Read the model definition and answer for the solid it produces. Units are mm, in the model's axes. A direction names the side the tool comes from. Give positions to 0.01 mm unless a question says otherwise; leave off trailing zeros. Loops run counter-clockwise (first coordinate to the right, second up) from the corner with the lowest first, then second, coordinate; pieces in that order, holes last. Notation, with made-up numbers: (-20, 48.25) - (16, 48.25) arc R26 ccw to (16, 80.25) - close; hole circle Ø7 at (-8.75, 86.5). An arc over 180 degrees is marked (long way). Use a Markdown table: item, result. Add a question column.
Item 1: For a pull along Y with two mould halves and no side action, classify faces 4 (the face through (12, 0, 26)), 5 (the face through (4.87, -6.51, 14.34)), 6 (the face through (-3.3, -0.6, 14.3)) as +Y half, -Y half, draft (parallel to the pull), parting line (faces both ways), or undercut.
Item 2: Which of the six approach directions +Z, -Z, +X, -X, +Y, -Y give full straight-line access (tool end or side, diameter ignored) to faces 1 (the face through (4.87, 8.49, 14.34)), 2 (the face through (15, 0, -12)), 3 (the face through (5, -7, 26))?
Item 3: A cutting plane is placed at B-B (x = 12.5). Determine the outline of the cut face in (y, z).
Item 4: Each of these flat-tipped pins is pushed along its axis until it touches: P1, Ø2, axis at x = -2.5, y = 4.5, coming from the +Z side; P2, Ø3, axis at y = 1, z = 17.5, coming from the -X side; P3, Ø8, axis at y = -8, z = 12.5, coming from the +X side. Where does it stop, or does it pass through?
Item 5: A cutting plane is placed at C-C (z = -14.5). Determine the outline of the cut face in (x, y).
Item 6: A cutting plane is placed at A-A (z = 8.5). Determine the outline of the cut face in (x, y), plus the area to 3 significant figures.
Item 7: Consider probe 1 along X at (y, z) = (6.75, -9.5); probe 2 along Y at (x, z) = (-4.25, -2.5); probe 3 along Z at (x, y) = (2.25, -7.25). Determine where each line is inside the solid, lowest interval first. Write a range as [from, to].
Item 8: A cutting plane is placed at D-D (y = 0). Determine the outline of the cut face in (x, z), plus the area to 3 significant figures.
from build123d import *

# Parameters (mm, degrees)
SKETCH1_W           = 26
SKETCH1_H           = 21
SKETCH1_W_2         = 20
SKETCH1_H_2         = 15
BOSS_EXTRUDE1_DEPTH = 25
SKETCH2_W           = 26
SKETCH2_H           = 21
BOSS_EXTRUDE2_DEPTH = 3
SKETCH3_R           = 1
BOSS_EXTRUDE3_DEPTH = 23


with BuildPart() as part:
    # Sketch1 → Boss-Extrude1 (new body)
    with BuildSketch(Plane.XY):
        with Locations((5, 0)):
            Rectangle(SKETCH1_W, SKETCH1_H)
        with Locations((5, 0)):
            Rectangle(SKETCH1_W_2, SKETCH1_H_2, mode=Mode.SUBTRACT)
    extrude(amount=-BOSS_EXTRUDE1_DEPTH)

    # Sketch2 → Boss-Extrude2 (add)
    with BuildSketch(Plane.XY):
        with Locations((5, 0)):
            Rectangle(SKETCH2_W, SKETCH2_H)
    extrude(amount=BOSS_EXTRUDE2_DEPTH)

    # Sketch3 → Boss-Extrude3 (add)
    with BuildSketch(Plane.XY.offset(3)):
        with Locations((12.5, 0)):
            Circle(SKETCH3_R)
        with Locations((5, -7.5)):
            Circle(SKETCH3_R)
        with Locations((-2.5, 0)):
            Circle(SKETCH3_R)
        with Locations((5, 7.5)):
            Circle(SKETCH3_R)
    extrude(amount=BOSS_EXTRUDE3_DEPTH)


solid = part.part
Geometry says:
| question | item | result |
|---|---|---|
| 1 | face 4 | draft |
| 1 | face 5 | undercut |
| 1 | face 6 | parting line |
| 2 | face 1 | +Z |
| 2 | face 2 | -Z |
| 2 | face 3 | +Z, +X, -X, +Y, -Y |
| 3 | outline | (-10.5, -25) - (-7.5, -25) - (-7.5, 0) - (7.5, 0) - (7.5, -25) - (10.5, -25) - (10.5, 3) - (1, 3) - (1, 26) - (-1, 26) - (-1, 3) - (-10.5, 3) - close |
| 4 | P1 | z = 3 |
| 4 | P2 | x = -3.5 |
| 4 | P3 | x = 6 |
| 5 | outline | (-8, -10.5) - (18, -10.5) - (18, 10.5) - (-8, 10.5) - close; hole (-5, -7.5) - (15, -7.5) - (15, 7.5) - (-5, 7.5) - close |
| 6 | outline | circle Ø2 at (-2.5, 0); circle Ø2 at (5, -7.5); circle Ø2 at (5, 7.5); circle Ø2 at (12.5, 0) |
| 6 | area | 12.6 mm² |
| 7 | probe 1 | [-8, -5], [15, 18] |
| 7 | probe 2 | [-10.5, -7.5], [7.5, 10.5] |
| 7 | probe 3 | [0, 3] |
| 8 | outline | (-8, -25) - (-5, -25) - (-5, 0) - (15, 0) - (15, -25) - (18, -25) - (18, 3) - (13.5, 3) - (13.5, 26) - (11.5, 26) - (11.5, 3) - (-1.5, 3) - (-1.5, 26) - (-3.5, 26) - (-3.5, 3) - (-8, 3) - close |
| 8 | area | 320 mm² |
